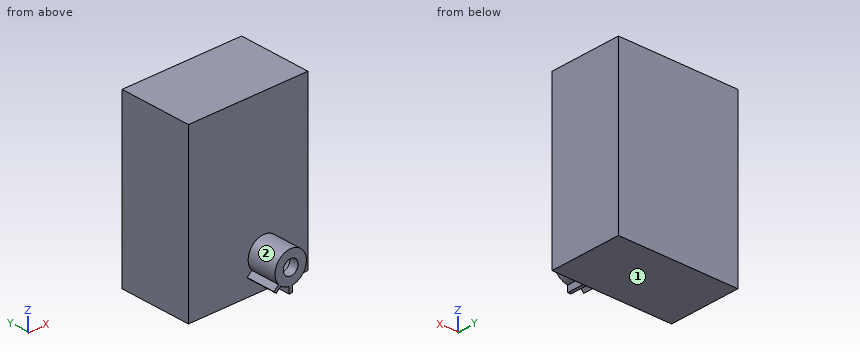
from build123d import *

# Parameters (mm, degrees)
SKETCH1_R           = 2.35
BOSS_EXTRUDE1_DEPTH = 9.3
SKETCH2_R           = 2.8
CUT_EXTRUDE1_DEPTH  = 6.5
SKETCH3_W           = 38
SKETCH3_H           = 53.5
BOSS_EXTRUDE2_DEPTH = 23


with BuildPart() as part:
    # Sketch1 → Boss-Extrude1 (new body)
    with BuildSketch(Plane(origin=(0, 0, 0), x_dir=(1, 0, 0), z_dir=(0, 1, 0))):
        with BuildLine():
            Line((-0.5, 7), (-0.5, 4.974937186))
            ThreePointArc((-0.5, 4.974937186), (-1.913417162, 4.619397663), (-3.164258429, 3.87136521))
            Line((-3.164258429, 3.87136521), (-4.583551024, 5.290657805))
            Line((-4.583551024, 5.290657805), (-5.290657805, 4.583551024))
            Line((-5.290657805, 4.583551024), (-3.87136521, 3.164258429))
            ThreePointArc((-3.87136521, 3.164258429), (1.913417162, -4.619397663), (0.5, 4.974937186))
            Line((0.5, 4.974937186), (0.5, 7))
            Line((0.5, 7), (-0.5, 7))
        make_face()
        with Locations(Location((0, 0, 0), (0, 0, 270))):
            Circle(SKETCH1_R, mode=Mode.SUBTRACT)
    extrude(amount=BOSS_EXTRUDE1_DEPTH)

    # Sketch2 → Cut-Extrude1 (cut)
    with BuildSketch(Plane(origin=(0, 9.3, 0), x_dir=(1, 0, 0), z_dir=(0, 1, 0))):
        with Locations(Location((0, 0, 0), (0, 0, 270))):
            Circle(SKETCH2_R)
    extrude(amount=-CUT_EXTRUDE1_DEPTH, mode=Mode.SUBTRACT)

    # Sketch3 → Boss-Extrude2 (add)
    with BuildSketch(Plane(origin=(0, 9.3, 0), x_dir=(1, 0, 0), z_dir=(0, 1, 0))):
        with Locations((-5, -16.75)):
            Rectangle(SKETCH3_W, SKETCH3_H)
    extrude(amount=BOSS_EXTRUDE2_DEPTH)


solid = part.part
Geometry: final body of the model. Coordinates: model frame, mm. Face numbers are marked on the shaded views. A direction names the side the tool comes from. Coordinates: 2 decimals unless noted, no trailing zeros. Order: outer loops, then holes, each group sorted by start corner. A loop starts at its lowest first (then second) coordinate and runs counter-clockwise, first axis right, second up. Notation, with made-up numbers: M -1,48.25 L 14,48.25 A27 ccw 14,81.25 Z; hole C 13,88.25 d9. An arc over 180 degrees is marked long. One line per question, with ' | ' between items. Start each with the question number.
Item 1: Cut plane B-B, the plane z = 0. Return the cut outline in (x, y), then the cut area to 3 significant figures.
Item 2: Cut plane A-A, the plane y = 5.5. Return the cut outline in (x, z).
Item 3: Cut plane C-C, the plane x = -7. Return the cut outline in (y, z).
Item 4: Cut plane D-D, the plane z = 36.5. Return the cut outline in (x, y).
Item 5: Set-up query: the marked faces 1 and 2. Return all of +Z, -Z, +X, -X, +Y, -Y with unobstructed straight access to the full face (end or side cutting, diameter ignored); none if empty.
Item 6: Ray query, probe 1 along Z at (x, y) = (0, 1); probe 2 along X at (y, z) = (2.1, 0); probe 3 along X at (y, z) = (7, 0). Return the intervals inside material, ascending. Write a range as [from, to].
Item 7: Pin query (flat end, axial travel): pin 1 Ø1 at (y, z) = (2.5, -6) entering from -X; pin 2 Ø3 at (x, z) = (-2, 12.5) entering from -Y; pin 3 Ø2 at (y, z) = (6.5, -5.5) entering from +X. Return the tip coordinate at first contact, or that it passes through.
A:
1) outline: M -24,9.3 L -5,9.3 L -5,0 L -2.35,0 L -2.35,2.8 L -2.8,2.8 L -2.8,9.3 L 2.8,9.3 L 2.8,2.8 L 2.35,2.8 L 2.35,0 L 5,0 L 5,9.3 L 14,9.3 L 14,32.3 L -24,32.3 Z | area: 917 mm2
2) outline: M -5.29,-4.58 L -4.58,-5.29 L -3.16,-3.87 A5 ccw -0.5,-4.97 L -0.5,-7 L 0.5,-7 L 0.5,-4.97 A5 ccw long -3.87,-3.16 Z; hole C 0,0 d5.6
3) outline: M 9.3,-10 L 32.3,-10 L 32.3,43.5 L 9.3,43.5 Z
4) outline: M -24,9.3 L 14,9.3 L 14,32.3 L -24,32.3 Z
5) face 1: -Z, +X, -X, +Y, -Y | face 2: -Y
6) probe 1: z = [-7, -2.35], [2.35, 5] | probe 2: x = [-5, -2.35], [2.35, 5] | probe 3: x = [-5, -2.8], [2.8, 5]
7) pin 1: stops at x = -0.5 | pin 2: stops at y = 9.3 | pin 3: stops at x = 2.18
